CAD build for the part. Positions are in the model's coordinates, mm. Face numbers are marked on the shaded views. A direction names the side the tool comes from. Give positions to 0.01 mm unless a question says otherwise; leave off trailing zeros. Write each loop counter-clockwise with the first axis right and the second up, starting at its lowest first coordinate (ties: lowest second). Pieces come first, ordered by that corner, then holes. Notation, with made-up numbers: (17, -36) - (42, -36) arc R22 cw to (42, -29) - close; hole circle Ø8 at (48.5, 67.25). An arc over 180 degrees is marked (long way). Answer as a JSON object with one key per item and string values.
from build123d import *

# Parameters (mm, degrees)
ESQUISSE1_W             = 53.5
ESQUISSE1_H             = 19.5
BOSS_EXTRU_1_DEPTH      = 1.5
ESQUISSE2_W             = 6
ESQUISSE2_H             = 4
BOSS_EXTRU_2_DEPTH      = 22.356
ESQUISSE3_W             = 1.5
ESQUISSE3_H             = 19.5
BOSS_EXTRU_3_DEPTH      = 6.144
ESQUISSE4_W             = 46
ESQUISSE4_H             = 1.5
BOSS_EXTRU_4_DEPTH      = 6.144
ENL_V_MAT_EXTRU_1_REACH = 42.803
ESQUISSE5_R             = 1.75
ESQUISSE6_R             = 1.75
ENL_V_MAT_EXTRU_2_DEPTH = 58.364917293


with BuildPart() as part:
    # Esquisse1 → Boss.-Extru.1 (new body)
    with BuildSketch(Plane(origin=(0, 0, 0), x_dir=(1, 0, 0), z_dir=(0, 1, 0))):
        Rectangle(ESQUISSE1_W, ESQUISSE1_H)
    extrude(amount=BOSS_EXTRU_1_DEPTH)

    # Esquisse2 → Boss.-Extru.2 (add)
    with BuildSketch(Plane(origin=(0, 1.5, 0), x_dir=(1, 0, 0), z_dir=(0, 1, 0))):
        with Locations((-23.75, -7.75)):
            Rectangle(ESQUISSE2_W, ESQUISSE2_H)
        with Locations((23.75, -7.75)):
            Rectangle(ESQUISSE2_W, ESQUISSE2_H)
    extrude(amount=BOSS_EXTRU_2_DEPTH)

    # Esquisse3 → Boss.-Extru.3 (add)
    with BuildSketch(Plane.XZ):
        with Locations((-23.75, 0)):
            Rectangle(ESQUISSE3_W, ESQUISSE3_H)
    boss_extru_3 = extrude(amount=BOSS_EXTRU_3_DEPTH)

    # Sym_trie1: Boss.-Extru.3 across plane
    add(boss_extru_3.mirror(Plane(origin=(0, 0, 0), x_dir=(0, 0, 1), z_dir=(1, 0, 0))))

    # Esquisse4 → Boss.-Extru.4 (add)
    with BuildSketch(Plane(origin=(0, 0, 0), x_dir=(-1, 0, 0), z_dir=(0, -1, 0))):
        with Locations((0, 9)):
            Rectangle(ESQUISSE4_W, ESQUISSE4_H)
    extrude(amount=BOSS_EXTRU_4_DEPTH)

    # Esquisse5 → Enl_v. mat.-Extru.1 (cut, up to next)
    with BuildSketch(Plane.XY.offset(9.75), mode=Mode.PRIVATE) as enl_v_mat_extru_1_sk1:
        with Locations((-23.75, 6.326)):
            Circle(ESQUISSE5_R)
    enl_v_mat_extru_1_tool1 = extrude(enl_v_mat_extru_1_sk1.sketch, amount=-ENL_V_MAT_EXTRU_1_REACH, mode=Mode.PRIVATE) & part.part
    # Esquisse5 → Enl_v. mat.-Extru.1 (cut, up to next)
    with BuildSketch(Plane.XY.offset(9.75), mode=Mode.PRIVATE) as enl_v_mat_extru_1_sk2:
        with Locations((-23.75, 16.486)):
            Circle(ESQUISSE5_R)
    enl_v_mat_extru_1_tool2 = extrude(enl_v_mat_extru_1_sk2.sketch, amount=-ENL_V_MAT_EXTRU_1_REACH, mode=Mode.PRIVATE) & part.part
    enl_v_mat_extru_1_1 = enl_v_mat_extru_1_tool1.solids().sort_by_distance((-23.75, 6.326, 9.75))[0]
    add(enl_v_mat_extru_1_1, mode=Mode.SUBTRACT)
    enl_v_mat_extru_1_2 = enl_v_mat_extru_1_tool2.solids().sort_by_distance((-23.75, 16.486, 9.75))[0]
    add(enl_v_mat_extru_1_2, mode=Mode.SUBTRACT)
    enl_v_mat_extru_1 = enl_v_mat_extru_1_1 + enl_v_mat_extru_1_2  # Enl_v. mat.-Extru.1 as one shape, for the pattern or mirror that repeats it

    # Sym_trie2: Enl_v. mat.-Extru.1 across plane
    add(enl_v_mat_extru_1.mirror(Plane(origin=(0, 0, 0), x_dir=(0, 0, 1), z_dir=(1, 0, 0))), mode=Mode.SUBTRACT)

    # Esquisse6 → Enl_v. mat.-Extru.2 (cut, through all)
    with BuildSketch(Plane.ZY.offset(24.5)):
        with Locations((6.678, -3.072)):
            Circle(ESQUISSE6_R)
    extrude(amount=-ENL_V_MAT_EXTRU_2_DEPTH, mode=Mode.SUBTRACT)


solid = part.part
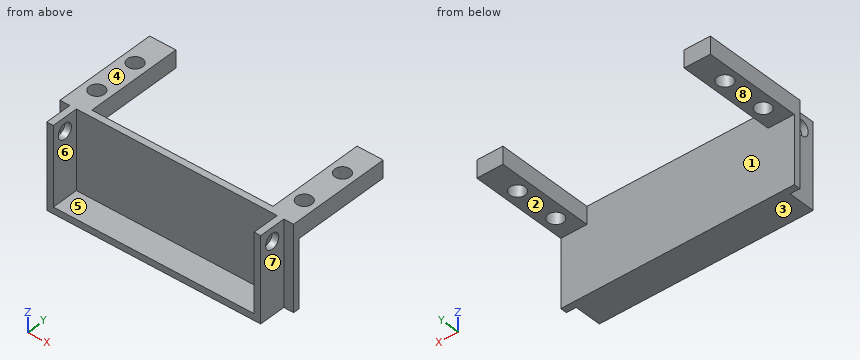
(1) Saw through at B-B, the plane x = -23.75. Give the cut face in (y, z).
Answer key:
{"outline": "(-6.14, -9.75) - (1.5, -9.75) - (1.5, 5.75) - (4.58, 5.75) - (4.58, 9.75) - (-6.14, 9.75) - close; (8.08, 5.75) - (14.74, 5.75) - (14.74, 9.75) - (8.08, 9.75) - close; (18.24, 5.75) - (23.86, 5.75) - (23.86, 9.75) - (18.24, 9.75) - close; hole circle Ø3.5 at (-3.07, 6.68)"}
(2) Flat gauge pins, fed straight in: P1, Ø1.1, axis at x = 26, z = 2, coming from the -Y side; P2, Ø5.5, axis at x = -23.75, y = 16.486, coming from the -Z side; P3, Ø3, axis at y = -3.5, z = -0.5, coming from the +X side. Where does each tip first touch, or does it go through?
Answer key:
{"P1": "stops at y = 0", "P2": "stops at z = 5.75", "P3": "stops at x = 24.5"}
(3) Probe L1, parallel to X at y = -1, z = -3.75; L2, parallel to Y at x = 23.75, z = 7; L3, parallel to Y at x = 15, z = -0.75. List the from-to ranges inside material, lowest first. Write a range as [from, to].
Answer key:
{"L1": "x = [-24.5, -23], [23, 24.5]", "L2": "y = [-6.14, -4.79], [-1.35, 4.58], [8.08, 14.74], [18.24, 23.86]", "L3": "y = [0, 1.5]"}
(4) Saw through at A-A, the plane y = 10.75. Give the cut face in (x, z).
Answer key:
{"outline": "(-26.75, 5.75) - (-20.75, 5.75) - (-20.75, 9.75) - (-26.75, 9.75) - close; (20.75, 5.75) - (26.75, 5.75) - (26.75, 9.75) - (20.75, 9.75) - close"}
(5) 3-axis set-ups, long thin cutter, end or side, ignore diameter. For the marked faces 1, 2, 3, 4 and 5: which of +Z, -Z, +X, -X, +Y, -Y reach the whole face in a straight line?
Answer key:
{"face 1": "-Z, +Y", "face 2": "-Z, +X, -X, +Y", "face 3": "-Z, +X, -X, +Y, -Y", "face 4": "+Z, +X, -X, +Y, -Y", "face 5": "+Z, -Y"}
(6) Saw through at C-C, the plane z = -6. Give the cut face in (x, y), and give its area (3 significant figures).
Answer key:
{"outline": "(-26.75, 0) - (-24.5, 0) - (-24.5, -6.14) - (-23, -6.14) - (-23, 0) - (23, 0) - (23, -6.14) - (24.5, -6.14) - (24.5, 0) - (26.75, 0) - (26.75, 1.5) - (-26.75, 1.5) - close", "area": "98.7 mm²"}
(7) Saw through at D-D, the plane y = 17.5. Give the cut face in (x, z).
Answer key:
{"outline": "(-26.75, 5.75) - (-25.18, 5.75) - (-25.18, 9.75) - (-26.75, 9.75) - close; (-22.32, 5.75) - (-20.75, 5.75) - (-20.75, 9.75) - (-22.32, 9.75) - close; (20.75, 5.75) - (22.32, 5.75) - (22.32, 9.75) - (20.75, 9.75) - close; (25.18, 5.75) - (26.75, 5.75) - (26.75, 9.75) - (25.18, 9.75) - close"}
(8) Pull direction X, two halves, no side cores. Call the marked faces 6, 7 and 8: pulls with the +X half, pulls with the -X half, needs draft (parallel to the pull), parting line crosses it, or undercut.
Answer key:
{"face 6": "undercut", "face 7": "pulls with the +X half", "face 8": "needs draft"}
